Check sheet for the modelled part. Datum: model origin and axes. Units: mm. Face numbers are marked on the shaded views. A direction names the side the tool comes from. Give positions to 0.01 mm unless a question says otherwise; leave off trailing zeros. Loops run counter-clockwise (first coordinate to the right, second up) from the corner with the lowest first, then second, coordinate; pieces in that order, holes last. Notation, with made-up numbers: (27, -9.75) - (50, -9.75) arc R16 ccw to (50, 4.25) - close; hole circle Ø5 at (-16.5, 57). An arc over 180 degrees is marked (long way). Use CSV: the item, a comma, the result in double quotes.
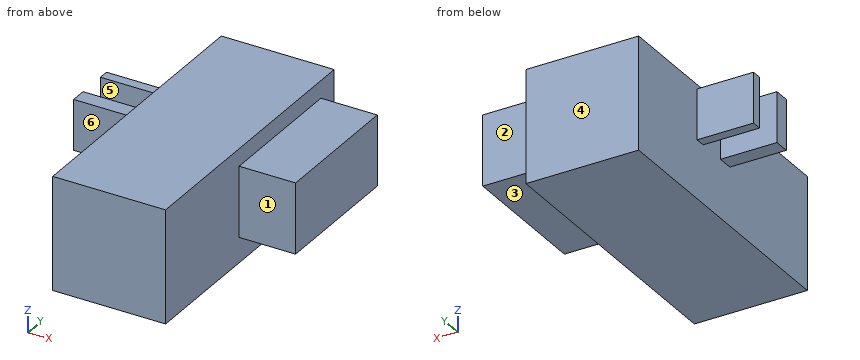
from build123d import *

# Parameters (mm, degrees)
F0_W     = 50.8
F0_H     = 50.8
F1_DEPTH = 127
F2_W     = 61.540618
F2_H     = 31.693089
F3_DEPTH = 25.4
F4_W     = 4.559308
F4_H     = 22.648551
F5_DEPTH = 25.4
F4_W_2   = 7.057599
F6_DEPTH = 25.4


with BuildPart() as f1:
    # F0 (on Front) → F1 (new body)
    with BuildSketch(Plane.XZ):
        with Locations((-10.617148, -0.824959)):
            Rectangle(F0_W, F0_H)
    extrude(amount=F1_DEPTH)

    # F2 (on face) → F3 (join, symmetric)
    with BuildSketch(Plane.YZ.offset(14.782852)):
        with Locations((-40.822573, 0.91443)):
            Rectangle(F2_W, F2_H)
    extrude(amount=F3_DEPTH, both=True)

    # F4 (on face) → F5 (join)
    with BuildSketch(Plane(origin=(-36.017148, 0, 0), x_dir=(0, -1, 0), z_dir=(-1, 0, 0))):
        with Locations((46.267241, 11.324275)):
            Rectangle(F4_W, F4_H)
    extrude(amount=F5_DEPTH)

    # F4 (on face) → F6 (join)
    with BuildSketch(Plane(origin=(-36.017148, 0, 0), x_dir=(0, -1, 0), z_dir=(-1, 0, 0))):
        with Locations((65.138158, 11.324275)):
            Rectangle(F4_W_2, F4_H)
    extrude(amount=F6_DEPTH)


solid = f1.part
1. Scan lines: line 1 along Y through (x, z) = (-49, 17.5); line 2 along X through (y, z) = (-56, -22.5); line 3 along Y through (x, z) = (27.5, 14). Record each from-to range of solid material in increasing order.
Completed:
line 1,"y = -68.67 to -61.61, -48.55 to -43.99"
line 2,"x = -36.02 to 14.78"
line 3,"y = -71.59 to -10.05"
2. Sectioned sample at B-B, the plane z = 15. Record the boundary of the cut face in (x, y).
Completed:
outline,"(-61.42, -68.67) - (-36.02, -68.67) - (-36.02, -127) - (14.78, -127) - (14.78, -71.59) - (40.18, -71.59) - (40.18, -10.05) - (14.78, -10.05) - (14.78, 0) - (-36.02, 0) - (-36.02, -43.99) - (-61.42, -43.99) - (-61.42, -48.55) - (-36.02, -48.55) - (-36.02, -61.61) - (-61.42, -61.61) - close"
3. Sectioned sample at C-C, the plane y = -38.5. Record the boundary of the cut face in (x, z).
Completed:
outline,"(-36.02, -26.22) - (14.78, -26.22) - (14.78, -14.93) - (40.18, -14.93) - (40.18, 16.76) - (14.78, 16.76) - (14.78, 24.58) - (-36.02, 24.58) - close"
4. Sectioned sample at D-D, the plane x = 18.5. Record the boundary of the cut face in (y, z), and give its area (3 significant figures).
Completed:
outline,"(-71.59, -14.93) - (-10.05, -14.93) - (-10.05, 16.76) - (-71.59, 16.76) - close"
area,"1,950 mm²"
5. Set-up check for the marked faces 1, 2 and 3: record each of +Z, -Z, +X, -X, +Y, -Y from which the full face is reachable in a straight line by a thin tool's end or side.
Completed:
face 1,"+Z, -Z, +X, -Y"
face 2,"+Z, -Z, +X, +Y"
face 3,"-Z, +X, +Y, -Y"
6. Release check for a two-part mould opening along Y. For the marked faces 4, 5 and 6 record: released by +Y, released by -Y, zero draft, split by the parting line, or undercut.
Completed:
face 4,"released by +Y"
face 5,"undercut"
face 6,"released by -Y"
7. Sectioned sample at A-A, the plane x = -37.5. Record the boundary of the cut face in (y, z), and give its area (3 significant figures).
Completed:
outline,"(-68.67, 0) - (-61.61, 0) - (-61.61, 22.65) - (-68.67, 22.65) - close; (-48.55, 0) - (-43.99, 0) - (-43.99, 22.65) - (-48.55, 22.65) - close"
area,"263 mm²"
8. Go/stop test with flat-tipped pins: pin 1 Ø18 at (x, z) = (-48.5, 9.5) entering from -Y; pin 2 Ø12.5 at (x, z) = (34, 6) entering from -Y; pin 3 Ø5.5 at (x, y) = (-50.5, -64.5) entering from +Z. Record where each tip stops, or that it passes through.
Completed:
pin 1,"stops at y = -68.67"
pin 2,"stops at y = -71.59"
pin 3,"stops at z = 22.65"
